Check sheet for the modelled part. Datum: model origin and axes. Units: mm. A direction names the side the tool comes from. Round coordinates to 2 decimals unless told otherwise and drop trailing zeros. Loops run counter-clockwise (first coordinate to the right, second up) from the corner with the lowest first, then second, coordinate; pieces in that order, holes last. Notation, with made-up numbers: (-0.75, 59.5) -> (47.25, 59.5) arc R21 cw to (47.25, 94.5) -> close; hole circle Ø5 at (72, 82). An arc over 180 degrees is marked (long way). One line per question, with ' | ' between items.
```python
from build123d import *

# Parameters (mm, degrees)
SKETCH_1_R      = 1.5
SKETCH_1_R_2    = 75
EXTRUDE_1_DEPTH = 6


with BuildPart() as part:
    # 草图1 → 凸台-拉伸1 (new body)
    with BuildSketch(Plane(origin=(0, 0, 0), x_dir=(1, 0, 0), z_dir=(0, 1, 0))):
        with BuildLine():
            Line((-128, 125.225), (-17.78, 125.225))
            Line((-17.78, 125.225), (-17.78, 105.225))
            Line((-17.78, 105.225), (-15, 105.225))
            Line((-15, 105.225), (-11.5, 105.225))
            ThreePointArc((-11.5, 105.225), (-10, 103.725), (-8.5, 105.225))
            Line((-8.5, 105.225), (-5, 105.225))
            Line((-5, 105.225), (-2.22, 105.225))
            Line((-2.22, 105.225), (-2.22, 125.225))
            Line((-2.22, 125.225), (108, 125.225))
            Line((108, 125.225), (108, 17.78))
            Line((108, 17.78), (88, 17.78))
            Line((88, 17.78), (88, 15))
            Line((88, 15), (88, 11.5))
            ThreePointArc((88, 11.5), (86.5, 10), (88, 8.5))
            Line((88, 8.5), (88, 5))
            Line((88, 5), (88, 2.22))
            Line((88, 2.22), (108, 2.22))
            Line((108, 2.22), (108, -105.225))
            Line((108, -105.225), (-2.22, -105.225))
            Line((-2.22, -105.225), (-2.22, -85.225))
            Line((-2.22, -85.225), (-5, -85.225))
            Line((-5, -85.225), (-8.5, -85.225))
            ThreePointArc((-8.5, -85.225), (-10, -83.725), (-11.5, -85.225))
            Line((-11.5, -85.225), (-15, -85.225))
            Line((-15, -85.225), (-17.78, -85.225))
            Line((-17.78, -85.225), (-17.78, -105.225))
            Line((-17.78, -105.225), (-128, -105.225))
            Line((-128, -105.225), (-128, 2.22))
            Line((-128, 2.22), (-108, 2.22))
            Line((-108, 2.22), (-108, 5))
            Line((-108, 5), (-108, 8.5))
            ThreePointArc((-108, 8.5), (-106.5, 10), (-108, 11.5))
            Line((-108, 11.5), (-108, 15))
            Line((-108, 15), (-108, 17.78))
            Line((-108, 17.78), (-128, 17.78))
            Line((-128, 17.78), (-128, 125.225))
        make_face()
        with Locations(Location((-108, 105.225, 0), (0, 0, 270))):
            Circle(SKETCH_1_R, mode=Mode.SUBTRACT)
        with Locations(Location((-59, 105.225, 0), (0, 0, 270))):
            Circle(SKETCH_1_R, mode=Mode.SUBTRACT)
        with Locations(Location((39, 105.225, 0), (0, 0, 270))):
            Circle(SKETCH_1_R, mode=Mode.SUBTRACT)
        with Locations(Location((88, 105.225, 0), (0, 0, 270))):
            Circle(SKETCH_1_R, mode=Mode.SUBTRACT)
        with Locations(Location((-108, -85.225, 0), (0, 0, 270))):
            Circle(SKETCH_1_R, mode=Mode.SUBTRACT)
        with Locations(Location((-59, -85.225, 0), (0, 0, 270))):
            Circle(SKETCH_1_R, mode=Mode.SUBTRACT)
        with Locations(Location((39, -85.225, 0), (0, 0, 270))):
            Circle(SKETCH_1_R, mode=Mode.SUBTRACT)
        with Locations(Location((88, -85.225, 0), (0, 0, 270))):
            Circle(SKETCH_1_R, mode=Mode.SUBTRACT)
        with Locations(Location((-10, 10, 0), (0, 0, 270))):
            Circle(SKETCH_1_R_2, mode=Mode.SUBTRACT)
    extrude(amount=EXTRUDE_1_DEPTH)


solid = part.part
```
(1) Go/stop test with flat-tipped pins: pin 1 (3 mm diameter, centred on x = -15.5, y = 4, fed in from -Z) (3 decimals); pin 2 (3 mm diameter, centred on y = 3, z = -5, fed in from -X). Record where each tip stops, or that it passes through.
Answer:
pin 1: stops at z = -105.225 | pin 2: stops at x = -108
(2) Set-up check for faces 4 (the face through (88, 3, -15)), 5 (the face through (-17.78, 3, 95)), 6 (the face through (-118, 3, -17.78)): record each of +Z, -Z, +X, -X, +Y, -Y from which the full face is reachable in a straight line by a thin tool's end or side.
Answer:
face 4: +X, +Y, -Y | face 5: +Z, +Y, -Y | face 6: -X, +Y, -Y
(3) Mould release check, pull along Z, two halves, no side actions. Record for faces 1 (the face through (-5, 3, -105.225)), 2 (the face through (-118, 3, -2.22)), 3 (the face through (-17.78, 3, -115)): +Z half, -Z half, draft (parallel to the pull), parting line (faces both ways), or undercut.
Answer:
face 1: -Z half | face 2: undercut | face 3: draft
(4) Sectioned sample at B-B, the plane x = -79.5. Record the cut outline in (y, z) (3 decimals).
Answer:
outline: (0, -125.225) -> (6, -125.225) -> (6, -38.191) -> (0, -38.191) -> close; (0, 18.191) -> (6, 18.191) -> (6, 105.225) -> (0, 105.225) -> close
(5) Sectioned sample at A-A, the plane z = 90. Record the cut outline in (x, y), and give its area (3 significant figures).
Answer:
outline: (-128, 0) -> (-17.78, 0) -> (-17.78, 6) -> (-128, 6) -> close; (-2.22, 0) -> (108, 0) -> (108, 6) -> (-2.22, 6) -> close | area: 1,320 mm2
(6) Sectioned sample at C-C, the plane y = 2.05. Count the separate pieces of the cut face and the enclosed holes in it, and give its area (3 significant figures).
Answer:
separate pieces: 1 | enclosed holes: 9 | area: 35,400 mm2
(7) Scan lines: probe 1 along X at (y, z) = (2, -10); probe 2 along X at (y, z) = (0.8, 87); probe 3 along X at (y, z) = (0.75, 86.5). Record each from-to range of solid material in increasing order.
Answer:
probe 1: x = -106.5 to -85, 65 to 86.5 | probe 2: x = -128 to -17.78, -2.22 to 108 | probe 3: x = -128 to -108.79, -107.21 to -59.79, -58.21 to -17.78, -2.22 to 38.21, 39.79 to 87.21, 88.79 to 108
